```python
from build123d import *

# Parameters (mm, degrees)
SKETCH1_W                = 56.03
SKETCH1_H                = 55.04
BOSS_EXTRUDE1_DEPTH      = 3
SKETCH2_R                = 6.19
SKETCH2_R_2              = 3.19
BOSS_EXTRUDE2_DEPTH      = 12
BOSS_EXTRUDE3_DEPTH      = 12
BOSS_EXTRUDE4_DEPTH      = 6
BOSS_EXTRUDE4_DEPTH_BACK = 6
SKETCH7_W                = 13
SKETCH7_H                = 11
FILLET1_R                = 5
SKETCH8_R                = 2.025
CUT_EXTRUDE3_DEPTH       = 13
CUT_EXTRUDE4_DEPTH       = 1.3
CUT_EXTRUDE4_DEPTH_BACK  = 1.3
CUT_EXTRUDE5_DEPTH       = 6
CUT_EXTRUDE5_DEPTH_BACK  = 3
SKETCH10_R               = 1.525
SKETCH11_R               = 3.309100225
CUT_EXTRUDE6_DEPTH       = 80.452894865
SKETCH12_W               = 7.33
SKETCH12_H               = 7.34
SKETCH12_W_2             = 5.68
CUT_EXTRUDE7_DEPTH       = 80.96100614


with BuildPart() as part:
    # Sketch1 → Boss-Extrude1 (new body)
    with BuildSketch(Plane(origin=(0, 0, 0), x_dir=(1, 0, 0), z_dir=(0, 1, 0))):
        with Locations((28.015, 27.52)):
            Rectangle(SKETCH1_W, SKETCH1_H)
    extrude(amount=BOSS_EXTRUDE1_DEPTH)

    # Sketch2 → Boss-Extrude2 (add)
    with BuildSketch(Plane(origin=(0, 3, 0), x_dir=(1, 0, 0), z_dir=(0, 1, 0))):
        with Locations(Location((28.015, 36.693201994, 0), (0, 0, 90))):
            Circle(SKETCH2_R)
        with Locations(Location((28.015, 36.693201994, 0), (0, 0, 270))):
            Circle(SKETCH2_R_2, mode=Mode.SUBTRACT)
    extrude(amount=BOSS_EXTRUDE2_DEPTH)

    # Sketch3 → Revolve1 (revolve)
    with BuildSketch(Plane(origin=(28.015, 0, 0), x_dir=(0, 0, -1), z_dir=(1, 0, 0))):
        Polygon((39.883201994, 15), (42.883201994, 15), (51.883201994, 3), (39.883201994, 3), align=None)
    revolve(axis=Axis((28.015, 15, -36.693201994), (0, -1, 0)))

    # Sketch5 → Boss-Extrude3 (add)
    with BuildSketch(Plane(origin=(0, 15, 0), x_dir=(1, 0, 0), z_dir=(0, 1, 0))):
        Polygon((28.015, 33.503201994), (24.778253514, 33.503201994), (24.778253514, 34.503201994), (31.698194277, 34.503201994), (31.698194277, 33.503201994), align=None)
    extrude(amount=-BOSS_EXTRUDE3_DEPTH)

    # Sketch7 → Boss-Extrude4 (add, two sides: drawn at the far end of the back side and taken through both)
    with BuildSketch(Plane(origin=(28.015, 0, 0), x_dir=(0, 0, -1), z_dir=(1, 0, 0)).offset(-BOSS_EXTRUDE4_DEPTH_BACK)):
        with Locations((28.003201994, 8.5)):
            Rectangle(SKETCH7_W, SKETCH7_H)
    extrude(amount=BOSS_EXTRUDE4_DEPTH + BOSS_EXTRUDE4_DEPTH_BACK)

    # Fillet1
    fillet1_edges = [part.edges().sort_by_distance(p)[0] for p in [
        (34.015, 14, -27.354384343),
        (22.015, 14, -27.354384343),
    ]]
    fillet(fillet1_edges, radius=FILLET1_R)

    # Sketch8 → Cut-Extrude3 (cut)
    with BuildSketch(Plane.XY.offset(-21.503201994)):
        with Locations((28.015, 8.53)):
            Circle(SKETCH8_R)
    extrude(amount=-CUT_EXTRUDE3_DEPTH, mode=Mode.SUBTRACT)

    # Sketch9 → Cut-Extrude4 (cut, two sides: drawn at the far end of the back side and taken through both)
    with BuildSketch(Plane.XY.offset(-28.003201994).offset(-CUT_EXTRUDE4_DEPTH_BACK)):
        Polygon((24.715, 10.435255888), (24.715, 15), (31.315, 15), (31.315, 10.435255888), (31.315, 6.624744112), (28.015, 4.719488223), (24.715, 6.624744112), align=None)
    extrude(amount=CUT_EXTRUDE4_DEPTH + CUT_EXTRUDE4_DEPTH_BACK, mode=Mode.SUBTRACT)

    # Sketch10 → Cut-Extrude5 (cut, two sides: drawn at the far end of the back side and taken through both)
    with BuildSketch(Plane(origin=(0, 3, 0), x_dir=(1, 0, 0), z_dir=(0, 1, 0)).offset(-CUT_EXTRUDE5_DEPTH_BACK)):
        with Locations(Location((28.015, 51.37, 0), (0, 0, 90))):
            Circle(SKETCH10_R)
        with Locations(Location((28.015, 3.67, 0), (0, 0, 90))):
            Circle(SKETCH10_R)
    extrude(amount=CUT_EXTRUDE5_DEPTH + CUT_EXTRUDE5_DEPTH_BACK, mode=Mode.SUBTRACT)

    # Sketch11 → Cut-Extrude6 (cut, through all)
    with BuildSketch(Plane(origin=(0, 3, 0), x_dir=(1, 0, 0), z_dir=(0, 1, 0))):
        with Locations((28.015, 51.37)):
            Circle(SKETCH11_R)
    extrude(amount=CUT_EXTRUDE6_DEPTH, mode=Mode.SUBTRACT)

    # Sketch12 → Cut-Extrude7 (cut, through all)
    with BuildSketch(Plane.XZ):
        with Locations((39.208604027, -51.37)):
            Rectangle(SKETCH12_W, SKETCH12_H)
        with Locations((17.65, -51.37)):
            Rectangle(SKETCH12_W_2, SKETCH12_H)
    extrude(amount=-CUT_EXTRUDE7_DEPTH, mode=Mode.SUBTRACT)


solid = part.part
```
Source: CAD feature listing. Evaluate the final solid. Frame: model axes, mm. A direction names the side the tool comes from. Coordinates: 2 decimals unless noted, no trailing zeros. Loops run counter-clockwise (first coordinate to the right, second up) from the corner with the lowest first, then second, coordinate; pieces in that order, holes last. Notation, with made-up numbers: (-14, 8.5) -> (4, 8.5) arc R17 ccw to (4, 18.5) -> close; hole circle Ø7 at (7.5, 51). An arc over 180 degrees is marked (long way). One line per item, written item: value. Start each with the question number.
Q1. Section query C-C, the plane z = -15. Return the cut outline in (x, y), and give its area (3 significant figures).
Q2. Mould query, pull axis Y, two halves, no side actions, for faces 6 (the face through (27.9, 3, -53.2)), 7 (the face through (56.03, 1, -27)), 8 (the face through (26.522, 9.899, -31.867)). Classes: pulls with the +Y half, pulls with the -Y half, needs draft (parallel to the pull), parting line crosses it, or undercut.
Q3. Line query: line 1 along X through (y, z) = (1.1, -51.37); line 2 along Y through (x, z) = (11, -24); line 3 along X through (y, z) = (6.75, -33). Output: solid intervals per line, ascending.
Q4. Contact query for flat-ended pins moving along their axis: P1, Ø8, axis at y = 11.5, z = -43, coming from the -X side; P2, Ø7.5, axis at x = 24.5, z = -51.5, coming from the +Y side; P3, Ø5, axis at x = 33, z = -8, coming from the +Y side. Output: stop coordinate, or through.
Q5. Section query A-A, the plane z = -3.67. Return the cut outline in (x, y).
Q6. Set-up query: faces 1 (the face through (32.511, 12.574, -25.883)), 2 (the face through (20.49, 1, -51)), 3 (the face through (28, 0, -28)), 4 (the face through (26.5, 1.5, -3.5)), 5 (the face through (28, 11, -29.303)). Return all of +Z, -Z, +X, -X, +Y, -Y with unobstructed straight access to the full face (end or side cutting, diameter ignored); none if empty.
Q7. Section query B-B, the plane x = 45.5. Return the cut outline in (y, z).
Results:
1. outline: (0, 0) -> (56.03, 0) -> (56.03, 3) -> (0, 3) -> close
1. area: 168 mm^2
2. face 6: pulls with the +Y half
2. face 7: needs draft
2. face 8: undercut
3. line 1: 0 to 14.81, 20.49 to 26.49, 29.54 to 35.54, 42.87 to 56.03
3. line 2: 0 to 3
3. line 3: 16.2 to 27.05, 28.98 to 39.83
4. P1: x = 17.44
4. P2: y = 7.96
4. P3: y = 3
5. outline: (0, 0) -> (26.49, 0) -> (26.49, 3) -> (0, 3) -> close; (29.54, 0) -> (56.03, 0) -> (56.03, 3) -> (29.54, 3) -> close
6. face 1: +Z, +X, +Y
6. face 2: -Z, +Y, -Y
6. face 3: +Z, -Z, +X, -X, -Y
6. face 4: +Y, -Y
6. face 5: +Y
7. outline: (0, -55.04) -> (3, -55.04) -> (3, 0) -> (0, 0) -> close
